```python
from build123d import *

# Parameters (mm, degrees)
F0_W      = 393.7
F0_H      = 381
F1_DEPTH  = 406.4
F2_W      = 381
F2_H      = 368.3
F3_DEPTH  = 400.05
F4_W      = 6.35
F4_H      = 368.3
F5_DEPTH  = 374.65
F6_W      = 101.6
F6_H      = 266.7
F7_DEPTH  = 6.35
F8_R      = 6.35
F9_DEPTH  = 6.35
F10_R     = 19.05
F11_DEPTH = 6.35
F12_R     = 19.05
F13_DEPTH = 6.35


with BuildPart() as f1:
    # F0 (on Top) → F1 (new body)
    with BuildSketch(Plane.XY):
        with Locations((-3.9738783777, -2.0195368604)):
            Rectangle(F0_W, F0_H)
    extrude(amount=-F1_DEPTH)

    # F2 (on face) → F3 (cut)
    with BuildSketch(Plane.XY):
        with Locations((-3.9738783777, -2.0195368604)):
            Rectangle(F2_W, F2_H)
    extrude(amount=-F3_DEPTH, mode=Mode.SUBTRACT)

    # F4 (on face) → F5 (join)
    with BuildSketch(Plane.XY):
        with Locations((-89.6988783777, -2.0195368604)):
            Rectangle(F4_W, F4_H)
    extrude(amount=-F5_DEPTH)

    # F6 (on face) → F7 (join)
    with BuildSketch(Plane.XY):
        with Locations((-143.6738783777, 48.7804631396)):
            Rectangle(F6_W, F6_H)
    extrude(amount=-F7_DEPTH)

    # F8 (on face) → F9 (cut)
    with BuildSketch(Plane.XY):
        with Locations((-143.3922201395, 159.0605080128)):
            Circle(F8_R)
    extrude(amount=-F9_DEPTH, mode=Mode.SUBTRACT)

    # F10 (on face) → F11 (cut)
    with BuildSketch(Plane.YZ.offset(192.8761216223)):
        with Locations((136.6306692362, -125.1103579998)):
            Circle(F10_R)
    extrude(amount=-F11_DEPTH, mode=Mode.SUBTRACT)

    # F12 (on face) → F13 (cut)
    with BuildSketch(Plane.YZ.offset(192.8761216223)):
        with Locations((137.2144669294, -50.3851957619)):
            Circle(F12_R)
    extrude(amount=-F13_DEPTH, mode=Mode.SUBTRACT)


solid = f1.part
```
CAD build for the part. Positions are in the model's coordinates, mm. A direction names the side the tool comes from. Round coordinates to 2 decimals unless told otherwise and drop trailing zeros. Order: outer loops, then holes, each group sorted by start corner. A loop starts at its lowest first (then second) coordinate and runs counter-clockwise, first axis right, second up.
Q1. Slice it at C-C (x = -120). Write the cut outline in (y, z), and give its area (3 significant figures).
Q2. Slice it at B-B (z = -198.5). Write the cut outline in (x, y).
Q3. Slice it at D-D (y = 95.5). Write the cut outline in (x, z), and give its area (3 significant figures).
Q4. Which spindle directions (+Z, -Z, +X, -X, +Y, -Y) get a long thin tool onto all of the face, cutting with end or side? Do faces 5 (the flat face through (-7, 188.48, -200)), 6 (the flat face through (-7, 182.13, -197)), 7 (the cylindrical face through (-140.46, 153.43, -3.13)), 8 (the cylindrical face through (189.746, 122.59, -112.235)), 9 (the flat face through (-200.824, -5, -200)). Say none if no direction does.
Q5. Wall check: L1, parallel to X at y = 107, z = -140; L2, parallel to Y at x = 59.5, z = -359.5; L3, parallel to X at y = -8, z = -381.5. Give the ranges that are in metal, low to high.
Q6. Drop a flat-ended pin along its axis: pin 1 (8 mm diameter, centred on x = -100.5, y = -98, fed in from +Z). Give the stop position or say it passes through.
Q7. Slice it at A-A (y = -96.5). Write the cut outline in (x, z).
Q8. Two-plate mould, pull along X, no slides. Class faces 1 (the flat face through (-194.474, -5, -197)), 2 (the flat face through (192.876, -5, -200)), 3 (the flat face through (-7, -192.52, -200)), 4 (the flat face through (-7, 1, -400.05)): pulls with the +X half, pulls with the -X half, needs draft (parallel to the pull), parting line crosses it, or undercut.
Results below:
1. outline: (-192.52, -406.4) - (188.48, -406.4) - (188.48, 0) - (-84.57, 0) - (-84.57, -6.35) - (182.13, -6.35) - (182.13, -400.05) - (-186.17, -400.05) - (-186.17, 0) - (-192.52, 0) - close
1. area: 9,190 mm2
2. outline: (-200.82, -192.52) - (192.88, -192.52) - (192.88, 188.48) - (-200.82, 188.48) - close; hole (-194.47, -186.17) - (-92.87, -186.17) - (-92.87, 182.13) - (-194.47, 182.13) - close; hole (-86.52, -186.17) - (186.53, -186.17) - (186.53, 182.13) - (-86.52, 182.13) - close
3. outline: (-200.82, -406.4) - (192.88, -406.4) - (192.88, 0) - (186.53, 0) - (186.53, -400.05) - (-194.47, -400.05) - (-194.47, -6.35) - (-92.87, -6.35) - (-92.87, -374.65) - (-86.52, -374.65) - (-86.52, 0) - (-200.82, 0) - close
3. area: 10,600 mm2
4. face 5: +Z, -Z, +X, -X, +Y
4. face 6: none
4. face 7: +Z
4. face 8: +X
4. face 9: +Z, -Z, -X, +Y, -Y
5. L1: x = -200.82 to -194.47, -92.87 to -86.52, 186.53 to 192.88
5. L2: y = -192.52 to -186.17, 182.13 to 188.48
5. L3: x = -200.82 to -194.47, 186.53 to 192.88
6. pin 1: stops at z = -400.05
7. outline: (-200.82, -406.4) - (192.88, -406.4) - (192.88, 0) - (186.53, 0) - (186.53, -400.05) - (-194.47, -400.05) - (-194.47, 0) - (-200.82, 0) - close; (-92.87, -374.65) - (-86.52, -374.65) - (-86.52, 0) - (-92.87, 0) - close
8. face 1: undercut
8. face 2: pulls with the +X half
8. face 3: needs draft
8. face 4: undercut
